Part model, mm, in its own coordinate system. A direction names the side the tool comes from. Round coordinates to 2 decimals unless told otherwise and drop trailing zeros. Write each loop counter-clockwise with the first axis right and the second up, starting at its lowest first coordinate (ties: lowest second). Pieces come first, ordered by that corner, then holes. Notation, with made-up numbers: (-18, 44.5) -> (3, 44.5) arc R27 ccw to (3, 70.5) -> close; hole circle Ø6 at (-6.75, 40.25). An arc over 180 degrees is marked (long way). Use CSV: the item, a comma, the result in double quotes. Start each with the question number.
```python
from build123d import *

# Parameters (mm, degrees)
SKETCH_1_R      = 1.5
SKETCH_1_W      = 6
SKETCH_1_H      = 6
EXTRUDE_1_DEPTH = 4
FILLET_1_R      = 3


with BuildPart() as part:
    # 草图1 → 凸台-拉伸1 (new body)
    # profile 1 of 4: a face of its own
    with BuildSketch(Plane(origin=(0, 0, 0), x_dir=(1, 0, 0), z_dir=(0, 1, 0))):
        Polygon((-116.482347914, -142.242252719), (-105.097347914, -142.242252719), (-105.097347914, -87.242252719), (-105.097347914, -32.242252719), (-30.097347914, -32.242252719), (-30.097347914, -87.242252719), (0.517652086, -87.242252719), (0.517652086, 7.757747281), (-116.482347914, 7.757747281), align=None)
        with Locations(Location((-83.482347914, -25.242252719, 0), (0, 0, 270))):
            Circle(SKETCH_1_R, mode=Mode.SUBTRACT)
        with Locations(Location((-23.482347914, -25.242252719, 0), (0, 0, 270))):
            Circle(SKETCH_1_R, mode=Mode.SUBTRACT)
    # profile 2 of 4: a face of its own
    with BuildSketch(Plane(origin=(0, 0, 0), x_dir=(1, 0, 0), z_dir=(0, 1, 0))):
        with BuildLine():
            Line((0.517652086, -87.242252719), (-30.097347914, -87.242252719))
            Line((-30.097347914, -87.242252719), (-30.097347914, -102.242252719))
            Line((-30.097347914, -102.242252719), (-24.982347914, -102.242252719))
            Line((-24.982347914, -102.242252719), (-24.982347914, -97.242252719))
            ThreePointArc((-24.982347914, -97.242252719), (-23.482347914, -95.742252719), (-21.982347914, -97.242252719))
            Line((-21.982347914, -97.242252719), (-21.982347914, -102.242252719))
            Line((-21.982347914, -102.242252719), (-16.982347914, -102.242252719))
            Line((-16.982347914, -102.242252719), (-16.982347914, -97.242252719))
            ThreePointArc((-16.982347914, -97.242252719), (-15.482347914, -95.742252719), (-13.982347914, -97.242252719))
            Line((-13.982347914, -97.242252719), (-13.982347914, -102.242252719))
            Line((-13.982347914, -102.242252719), (-8.982347914, -102.242252719))
            Line((-8.982347914, -102.242252719), (-8.982347914, -97.242252719))
            ThreePointArc((-8.982347914, -97.242252719), (-7.482347914, -95.742252719), (-5.982347914, -97.242252719))
            Line((-5.982347914, -97.242252719), (-5.982347914, -102.242252719))
            Line((-5.982347914, -102.242252719), (-0.982347914, -102.242252719))
            Line((-0.982347914, -102.242252719), (-0.982347914, -97.242252719))
            ThreePointArc((-0.982347914, -97.242252719), (-0.543008086, -96.181592547), (0.517652086, -95.742252719))
            Line((0.517652086, -95.742252719), (0.517652086, -87.242252719))
        make_face()
    # profile 3 of 4: a face of its own
    with BuildSketch(Plane(origin=(0, 0, 0), x_dir=(1, 0, 0), z_dir=(0, 1, 0))):
        with BuildLine():
            Line((-88.097347914, -142.242252719), (-80.097347914, -142.242252719))
            Line((-80.097347914, -142.242252719), (-80.097347914, -113.742252719))
            Line((-80.097347914, -113.742252719), (-80.097347914, -113.242252719))
            Line((-80.097347914, -113.242252719), (-86.097347914, -113.242252719))
            Line((-86.097347914, -113.242252719), (-86.097347914, -107.242252719))
            Line((-86.097347914, -107.242252719), (-80.097347914, -107.242252719))
            Line((-80.097347914, -107.242252719), (-80.097347914, -87.242252719))
            Line((-80.097347914, -87.242252719), (-105.097347914, -87.242252719))
            Line((-105.097347914, -87.242252719), (-105.097347914, -142.242252719))
            Line((-105.097347914, -142.242252719), (-99.097347914, -142.242252719))
            Line((-99.097347914, -142.242252719), (-99.097347914, -127.242252719))
            ThreePointArc((-99.097347914, -127.242252719), (-97.597347914, -125.742252719), (-96.097347914, -127.242252719))
            Line((-96.097347914, -127.242252719), (-96.097347914, -142.242252719))
            Line((-96.097347914, -142.242252719), (-91.097347914, -142.242252719))
            Line((-91.097347914, -142.242252719), (-91.097347914, -127.242252719))
            ThreePointArc((-91.097347914, -127.242252719), (-89.597347914, -125.742252719), (-88.097347914, -127.242252719))
            Line((-88.097347914, -127.242252719), (-88.097347914, -142.242252719))
        make_face()
        with Locations(Location((-102.597347914, -117.242252719, 0), (0, 0, 270))):
            Circle(SKETCH_1_R, mode=Mode.SUBTRACT)
        with Locations(Location((-84.897347914, -117.242252719, 0), (0, 0, 270))):
            Circle(SKETCH_1_R, mode=Mode.SUBTRACT)
        with Locations(Location((-88.387347914, -92.242252719, 0), (0, 0, 270))):
            Circle(SKETCH_1_R, mode=Mode.SUBTRACT)
    # profile 4 of 4: a face of its own
    with BuildSketch(Plane(origin=(0, 0, 0), x_dir=(1, 0, 0), z_dir=(0, 1, 0))):
        with Locations((-83.097347914, -110.242252719)):
            Rectangle(SKETCH_1_W, SKETCH_1_H)
        with Locations(Location((-83.097347914, -110.242252719, 0), (0, 0, 270))):
            Circle(SKETCH_1_R, mode=Mode.SUBTRACT)
    extrude(amount=EXTRUDE_1_DEPTH)

    # 圆角1
    fillet_1_edges = [part.edges().sort_by_distance(p)[0] for p in [
        (-30.097347914, 2, 102.242252719),
        (-30.097347914, 2, 32.242252719),
        (-105.097347914, 2, 32.242252719),
        (-105.097347914, 2, 87.242252719),
        (-80.097347914, 2, 87.242252719),
        (-116.482347914, 2, 142.242252719),
        (-116.482347914, 2, -7.757747281),
        (0.517652086, 2, -7.757747281),
    ]]
    fillet(fillet_1_edges, radius=FILLET_1_R)


solid = part.part
```
1. Band-saw the part on C-C (y = 1.2). Give the number of separate pieces and of enclosed holes in the cut face, then the cut area to 3 significant figures.
2. Drill centre lines: line 1 along Z through (x, y) = (-102.5, 0.7); line 2 along X through (y, z) = (2.9, 133.5); line 3 along X through (y, z) = (3.1, 47). Where is each one in solid material? Low to high. Write a range as [from, to].
3. Band-saw the part on B-B (x = -57.5). List the corners of the cut face in (y, z), then the cut area to 3 significant figures.
4. Which spindle directions (+Z, -Z, +X, -X, +Y, -Y) get a long thin tool onto all of the face, cutting with end or side? Do faces 5 (the flat face through (-57, 2, -7.758)), 6 (the cylindrical face through (-104.195, 2.028, 86.387)), 7 (the flat face through (-13.982, 2, 100)), 8 (the flat face through (-4, 2, 102.242)), 9 (the cylindrical face through (-0.34, 2.03, -6.86)). Say none if no direction does.
5. Pull direction Z, two halves, no side cores. Call faces 1 (the cylindrical face through (-101.333, 1.972, 118.049)), 2 (the cylindrical face through (-23.515, 1.972, 95.743)), 3 (the cylindrical face through (-115.58, 2.03, -6.9)), 4 (the flat face through (-24.982, 2, 100)): released by +Z, released by -Z, zero draft, split by the parting line, or undercut.
6. Flat gauge pins, fed straight in: pin 1 (0.6 mm diameter, centred on x = -26.5, y = 2.5, fed in from +Z); pin 2 (2.5 mm diameter, centred on x = -88.39, z = 92.24, fed in from +Y); pin 3 (2 mm diameter, centred on y = 2.5, z = 124.5, fed in from +X). Where does each tip first touch, or does it go through?
7. Band-saw the part on A-A (z = 38). List the corners of the cut face in (x, y).
Answers below:
1,separate pieces,"1"
1,enclosed holes,"6"
1,area,"9,240 mm^2"
2,line 1,"z = [-7.76, 32.27], [87.22, 115.75], [118.74, 142.24]"
2,line 2,"x = [-116.48, -99.1], [-96.1, -91.1], [-88.1, -80.1]"
2,line 3,"x = [-116.48, -105.1], [-30.1, 0.52]"
3,outline,"(0, -7.76) -> (4, -7.76) -> (4, 32.24) -> (0, 32.24) -> close"
3,area,"160 mm^2"
4,face 5,"-Z, +X, -X, +Y, -Y"
4,face 6,"+Y, -Y"
4,face 7,"+Z, +Y, -Y"
4,face 8,"+Z, +X, +Y, -Y"
4,face 9,"-Z, +X, +Y, -Y"
5,face 1,"undercut"
5,face 2,"released by +Z"
5,face 3,"released by -Z"
5,face 4,"zero draft"
6,pin 1,"stops at z = 102.24"
6,pin 2,"passes through"
6,pin 3,"stops at x = -80.1"
7,outline,"(-116.48, 0) -> (-105.1, 0) -> (-105.1, 4) -> (-116.48, 4) -> close; (-30.1, 0) -> (0.52, 0) -> (0.52, 4) -> (-30.1, 4) -> close"
